```python
from build123d import *

# Parameters (mm, degrees)
F0_W     = 4.7
F0_H     = 5
F1_DEPTH = 6
F2_R     = 2
F3_DEPTH = 5
F4_W     = 4.7
F4_H     = 1.9
F5_DEPTH = 6


with BuildPart() as f1:
    # F0 (on Top) → F1 (new body)
    with BuildSketch(Plane.XY):
        with Locations((-58.38673, 37.343877)):
            Rectangle(F0_W, F0_H)
    extrude(amount=F1_DEPTH)

    # F2 (on face) → F3 (cut)
    with BuildSketch(Plane.XY.offset(6)):
        with Locations((-58.38673, 37.343877)):
            Circle(F2_R)
    extrude(amount=-F3_DEPTH, mode=Mode.SUBTRACT)

    # F4 (on face) → F5 (join)
    with BuildSketch(Plane(origin=(0, 0, 0), x_dir=(1, 0, 0), z_dir=(0, 0, -1))):
        with Locations((-58.38673, -37.343877)):
            Rectangle(F4_W, F4_H)
    extrude(amount=F5_DEPTH)


solid = f1.part
```
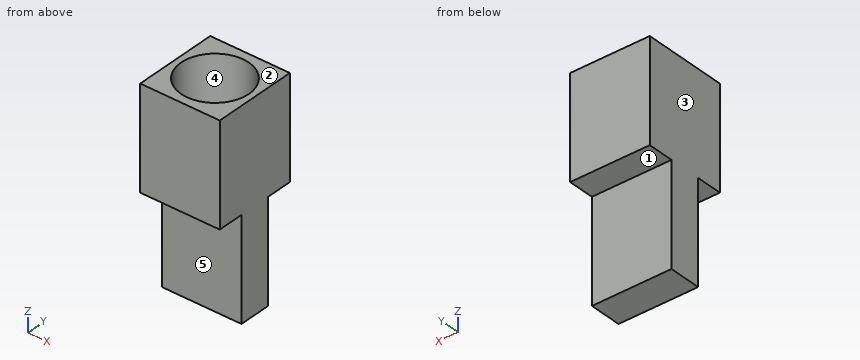
For this review, take the finished solid that the model builds, in its own axes (mm). Face numbers are marked on the shaded views. A direction names the side the tool comes from. Give positions to 0.01 mm unless a question says otherwise; leave off trailing zeros. Order: outer loops, then holes, each group sorted by start corner. A loop starts at its lowest first (then second) coordinate and runs counter-clockwise, first axis right, second up.
1) Take a section at B-B (y = 38.5). Give the boundary of the cut face in (x, z), then the cut area to 3 significant figures.
2) Take a section at C-C (z = 5). Give the boundary of the cut face in (x, y), then the cut area to 3 significant figures.
3) For the marked faces 1 and 2, list the 3-axis set-ups (+Z, -Z, +X, -X, +Y, -Y) from which the entire face can be reached by the end or side of a thin tool; tool diameter is ignored.
4) Take a section at A-A (x = -58.3). Give the boundary of the cut face in (y, z), then the cut area to 3 significant figures.
5) Wall thickness on line 1 (Z direction, x = -57.95, y = 36.6); line 2 (Y direction, x = -59.7, z = -1.5); line 3 (Y direction, x = -58.4, z = 4.75): over which ranges is each line inside the solid? List them lowest first.
6) Take a section at D-D (z = -4.75). Give the boundary of the cut face in (x, y), then the cut area to 3 significant figures.
7) The part is to be moulded in two halves that separate along X. For the marked faces 3, 4 and 5, say which applies: released by +X, released by -X, zero draft, split by the parting line, or undercut.
8) Insertion check: pin 1 (2 mm diameter, centred on x = -59, z = -2, fed in from +Y); pin 2 (0.5 mm diameter, centred on x = -58, y = 39, fed in from -Z). Each pin has a flat end and moves straight along its axis. Give the tip position at first contact, or say it passes through.
Derived:
1. outline: (-60.74, 0) - (-56.04, 0) - (-56.04, 6) - (-56.75, 6) - (-56.75, 1) - (-60.02, 1) - (-60.02, 6) - (-60.74, 6) - close
1. area: 11.9 mm2
2. outline: (-60.74, 34.84) - (-56.04, 34.84) - (-56.04, 39.84) - (-60.74, 39.84) - close; hole circle Ø4 at (-58.39, 37.34)
2. area: 10.9 mm2
3. face 1: -Z, +X, -X, +Y
3. face 2: +Z, +X, -X, +Y, -Y
4. outline: (34.84, 0) - (36.39, 0) - (36.39, -6) - (38.29, -6) - (38.29, 0) - (39.84, 0) - (39.84, 6) - (39.34, 6) - (39.34, 1) - (35.35, 1) - (35.35, 6) - (34.84, 6) - close
4. area: 21.4 mm2
5. line 1: z = -6 to 1
5. line 2: y = 36.39 to 38.29
5. line 3: y = 34.84 to 35.34, 39.34 to 39.84
6. outline: (-60.74, 36.39) - (-56.04, 36.39) - (-56.04, 38.29) - (-60.74, 38.29) - close
6. area: 8.93 mm2
7. face 3: released by -X
7. face 4: undercut
7. face 5: zero draft
8. pin 1: stops at y = 38.29
8. pin 2: stops at z = 0
